Verification items for the finished model (mm, model axes). Coordinates: 2 decimals unless noted, no trailing zeros. Order: outer loops, then holes, each group sorted by start corner. A loop starts at its lowest first (then second) coordinate and runs counter-clockwise, first axis right, second up. Notation, with made-up numbers: (22.5, 2.25) -> (38.5, 2.25) arc R13 cw to (38.5, 23.25) -> close; hole circle Ø6 at (88, -7.75). An arc over 180 degrees is marked (long way). Write each question's results on one line, items separated by ' | '. Start each with the question number.
(1) Thickness scan on probe 1 along Y at (x, z) = (52, 2.7); probe 2 along X at (y, z) = (29.5, 0.75); probe 3 along Y at (x, z) = (12.5, 0.6). Record the ranges inside material, lowest first. Write a range as [from, to].
(2) Cross-section at A-A on z = 1.3. Enter the section's corners in (x, y).
(3) Cross-section at C-C on y = 78. Enter the section's corners in (x, z), and give its area (3 significant figures).
(4) Cross-section at B-B on x = 23. Enter the section's corners in (y, z), and give its area (3 significant figures).
(5) Go/stop test with flat-tipped pins: pin 1 (0.9 mm diameter, centred on x = 90, z = 2, fed in from -Y); pin 2 (1.5 mm diameter, centred on y = -9, z = 1, fed in from -X). Record where each tip stops, or that it passes through.
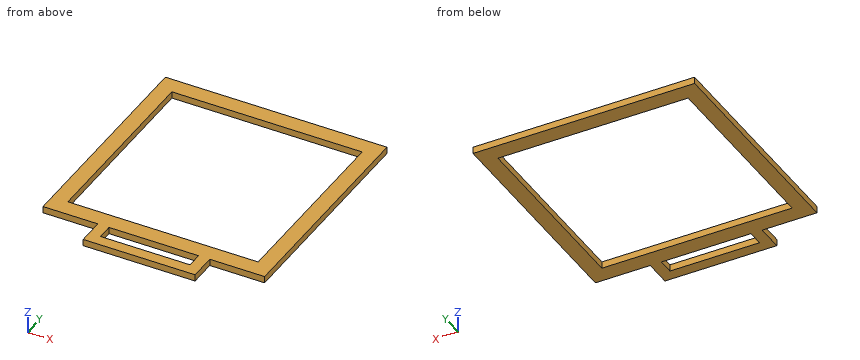
```python
from build123d import *

# Parameters (mm, degrees)
CROQUIS1_W              = 99
CROQUIS1_H              = 100
CROQUIS1_W_2            = 85
CROQUIS1_H_2            = 85
SALIENTE_EXTRUIR1_DEPTH = 3
SALIENTE_EXTRUIR2_DEPTH = 3


with BuildPart() as part:
    # Croquis1 → Saliente-Extruir1 (new body)
    with BuildSketch(Plane.XY):
        with Locations((49.5, 50)):
            Rectangle(CROQUIS1_W, CROQUIS1_H)
        with Locations((49.5, 50)):
            Rectangle(CROQUIS1_W_2, CROQUIS1_H_2, mode=Mode.SUBTRACT)
    extrude(amount=SALIENTE_EXTRUIR1_DEPTH)

    # Croquis2 → Saliente-Extruir2 (add)
    with BuildSketch(Plane.XY.offset(3)):
        Polygon((24.5, 0), (29.5, 0), (29.5, -7), (69.5, -7), (69.5, 0), (74.5, 0), (74.5, -12), (24.5, -12), align=None)
    extrude(amount=-SALIENTE_EXTRUIR2_DEPTH)


solid = part.part
```
Results are:
1) probe 1: y = [-12, -7], [0, 7.5], [92.5, 100] | probe 2: x = [0, 7], [92, 99] | probe 3: y = [0, 7.5], [92.5, 100]
2) outline: (0, 0) -> (24.5, 0) -> (24.5, -12) -> (74.5, -12) -> (74.5, 0) -> (99, 0) -> (99, 100) -> (0, 100) -> close; hole (7, 7.5) -> (92, 7.5) -> (92, 92.5) -> (7, 92.5) -> close; hole (29.5, -7) -> (69.5, -7) -> (69.5, 0) -> (29.5, 0) -> close
3) outline: (0, 0) -> (7, 0) -> (7, 3) -> (0, 3) -> close; (92, 0) -> (99, 0) -> (99, 3) -> (92, 3) -> close | area: 42.0 mm2
4) outline: (0, 0) -> (7.5, 0) -> (7.5, 3) -> (0, 3) -> close; (92.5, 0) -> (100, 0) -> (100, 3) -> (92.5, 3) -> close | area: 45.0 mm2
5) pin 1: stops at y = 0 | pin 2: stops at x = 24.5
